Geometry check sheet. Reference: drawing and pictorial views, mm from the part's lowest x, y, z. A direction names the side the tool comes from. Give positions to 0.01 mm unless a question says otherwise; leave off trailing zeros. Write each loop counter-clockwise with the first axis right and the second up, starting at its lowest first coordinate (ties: lowest second). Pieces come first, ordered by that corner, then holes. Notation, with made-up numbers: (14.5, 74.5) -> (50.5, 74.5) arc R26 cw to (50.5, 96.5) -> close; hole circle Ø8 at (-33.5, 3). An arc over 180 degrees is marked (long way). Use a Markdown table: item, result. Add a question column.
1. Cross-section at A-A (y = 29). Enter the section's corners in (x, z).
2. Scan lines: probe 1 along X at (y, z) = (26.5, 12.25); probe 2 along Y at (x, z) = (26.5, 9.5); probe 3 along Z at (x, y) = (48.5, 69.5). Record each from-to range of solid material in increasing order. Write a range as [from, to].
3. Gauge pin test, flat ends, axial feed: P1, Ø1.9, axis at x = 56, z = 2, coming from the +Y side; P2, Ø1.9, axis at y = 27.5, z = 2.5, coming from the +X side. Record the tip position at first contact, or that the pin passes through.
4. Cross-section at B-B (x = 37). Enter the section's corners in (y, z).
5. Cross-section at C-C (z = 7.5). Enter the section's corners in (x, y).
6. Set-up check for the marked faces 1 and 2: record each of +Z, -Z, +X, -X, +Y, -Y from which the full face is reachable in a straight line by a thin tool's end or side.
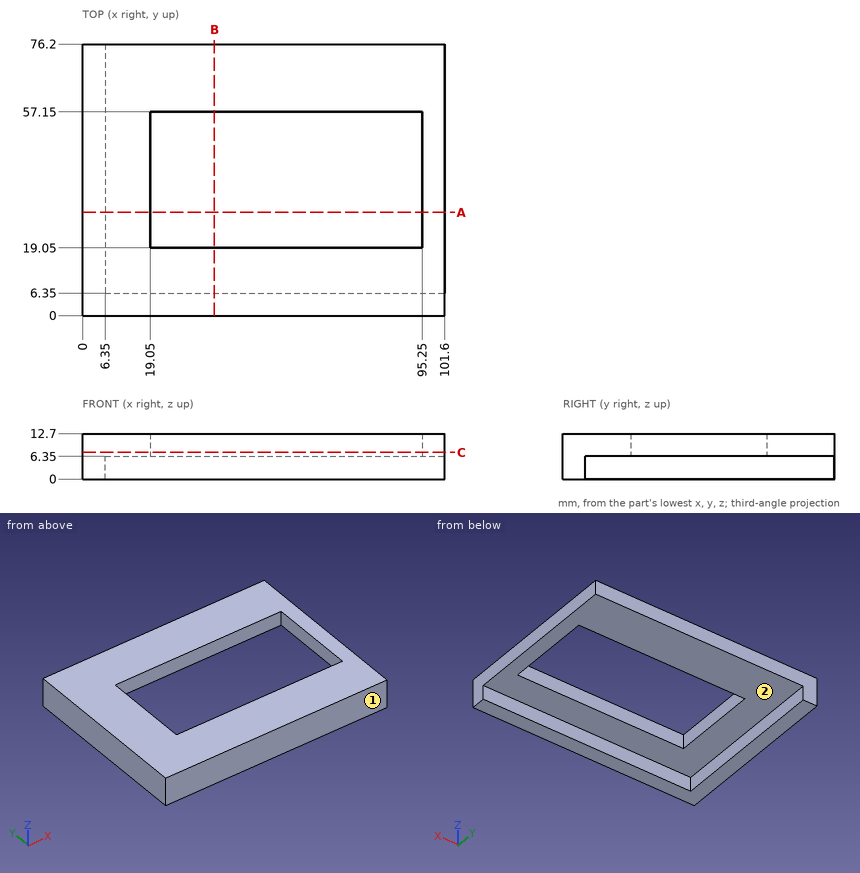
Worked answers:
| question | item | result |
|---|---|---|
| 1 | outline | (0, 0) -> (6.35, 0) -> (6.35, 6.35) -> (19.05, 6.35) -> (19.05, 12.7) -> (0, 12.7) -> close; (95.25, 6.35) -> (101.6, 6.35) -> (101.6, 12.7) -> (95.25, 12.7) -> close |
| 2 | probe 1 | x = [0, 19.05], [95.25, 101.6] |
| 2 | probe 2 | y = [0, 19.05], [57.15, 76.2] |
| 2 | probe 3 | z = [6.35, 12.7] |
| 3 | P1 | stops at y = 6.35 |
| 3 | P2 | stops at x = 6.35 |
| 4 | outline | (0, 0) -> (6.35, 0) -> (6.35, 6.35) -> (19.05, 6.35) -> (19.05, 12.7) -> (0, 12.7) -> close; (57.15, 6.35) -> (76.2, 6.35) -> (76.2, 12.7) -> (57.15, 12.7) -> close |
| 5 | outline | (0, 0) -> (101.6, 0) -> (101.6, 76.2) -> (0, 76.2) -> close; hole (19.05, 19.05) -> (95.25, 19.05) -> (95.25, 57.15) -> (19.05, 57.15) -> close |
| 6 | face 1 | +Z, -Z, +X, -X, -Y |
| 6 | face 2 | -Z, +X, +Y |
